from build123d import *

# Parameters (mm, degrees)
BOSS_EXTRUDE1_DEPTH      = 3
BOSS_EXTRUDE1_DEPTH_BACK = 7
FILLET1_R                = 1
SKETCH2_R                = 1.5
CUT_EXTRUDE1_DEPTH       = 22.698151839
CIRPATTERN1_COUNT        = 5


with BuildPart() as part:
    # Sketch1 → Boss-Extrude1 (new, two sides: drawn at the far end of the back side and taken through both)
    with BuildSketch(Plane(origin=(0, 0, 0), x_dir=(1, 0, 0), z_dir=(0, 1, 0)).offset(-BOSS_EXTRUDE1_DEPTH_BACK)):
        Polygon((-7.26542528, -10), (7.26542528, -10), (11.755705046, 3.819660113), (0, 12.360679775), (-11.755705046, 3.819660113), align=None)
    extrude(amount=BOSS_EXTRUDE1_DEPTH + BOSS_EXTRUDE1_DEPTH_BACK)

    # Fillet1
    fillet1_edges = [part.edges().sort_by_distance(p)[0] for p in [
        (9.510565163, -7, 3.090169944),
        (-9.510565163, 3, 3.090169944),
        (0, 3, 10),
        (9.510565163, 3, 3.090169944),
        (5.877852523, 3, -8.090169944),
        (-5.877852523, 3, -8.090169944),
        (5.877852523, -7, -8.090169944),
        (-5.877852523, -7, -8.090169944),
        (-9.510565163, -7, 3.090169944),
        (0, -7, 10),
    ]]
    fillet(fillet1_edges, radius=FILLET1_R)

    # Sketch2 → Cut-Extrude1 (cut, through all)
    with BuildSketch(Plane(origin=(-2.261652721, -1.093066116, 3.112897916), x_dir=(-0.824807817325119, 0.18732666439624865, -0.533479882737436), z_dir=(0.56541318031982, 0.2732665289126595, -0.7782244789883274))):
        with Locations(Location((0, 0, 0), (0, 0, 348.770538042))):
            Circle(SKETCH2_R)
    cut_extrude1 = extrude(amount=-CUT_EXTRUDE1_DEPTH, mode=Mode.SUBTRACT)

    # CirPattern1: Cut-Extrude1 ×5 about axis
    cirpattern1_axis = Axis((0, 0, 0), (0, 1, 0))
    for i in range(1, CIRPATTERN1_COUNT):
        add(cut_extrude1.rotate(cirpattern1_axis, i * 360 / CIRPATTERN1_COUNT), mode=Mode.SUBTRACT)


solid = part.part
Geometry: final body of the model. Coordinates: model frame, mm. A direction names the side the tool comes from. Coordinates: 2 decimals unless noted, no trailing zeros. Order: outer loops, then holes, each group sorted by start corner. A loop starts at its lowest first (then second) coordinate and runs counter-clockwise, first axis right, second up.
(1) Access query for faces 1 (the face through (-0.021, -1.073, -3.853)), 2 (the face through (9.27, -6.7, 2.91)). Directions: +Z, -Z, +X, -X, +Y, -Y. A direction counts if a zero-diameter tool reaches every point of the face in a straight line with its end or side. Return the directions, or none.
(2) Material intervals for probe 1 along Z at (x, y) = (4.5, -1.25); probe 2 along X at (y, z) = (-2.25, 3.25); probe 3 along Y at (x, z) = (-8, -2.5), sorted ascending.
(3) First-contact query: pin 1 (5 mm diameter, centred on y = -2.5, z = 5, fed in from +X); pin 2 (1.5 mm diameter, centred on y = 1, z = -4, fed in from -X); pin 3 (1 mm diameter, centred on y = -1, z = 6.5, fed in from -X); pin 4 (1 mm diameter, centred on x = 7.5, y = 2, fed in from -Z). Flat tips, straight axial feed; report the tip coordinate or a pass-through.
(4) Section query B-B (y = -0.75). State how many separate pieces and enclosed holes the cut face has, plus the area to 3 significant figures.
(5) Draft query along Z for faces 3 (the face through (-9.208, 2.699, 3.099)), 4 (the face through (4.875, -3.751, 6.157)), 5 (the face through (5.63, 2.7, -7.92)). Return one class per face: pulls with the +Z half, pulls with the -Z half, needs draft (parallel to the pull), parting line crosses it, or undercut.
(6) Section query A-A (y = 1). Return the cut outline in (x, z), plus the area to 3 significant figures.
Solution:
1. face 1: none
1. face 2: +Z, +X, -Y
2. probe 1: z = -9.09 to -3.02, 0.11 to 3.71, 7.68 to 10
2. probe 2: x = -9.46 to -3.92, -1.51 to 1.51, 3.92 to 9.46
2. probe 3: y = -7 to -3.94, -0.82 to 3
3. pin 1: stops at x = 9.7
3. pin 2: stops at x = -11.76
3. pin 3: stops at x = -8.57
3. pin 4: stops at z = -7.27
4. separate pieces: 1
4. enclosed holes: 5
4. area: 318 mm2
5. face 3: pulls with the +Z half
5. face 4: undercut
5. face 5: pulls with the -Z half
6. outline: (-11.76, -3.82) - (0, -12.36) - (11.76, -3.82) - (7.27, 10) - (-7.27, 10) - close
6. area: 363 mm2
